```python
from build123d import *

# Parameters (mm, degrees)
F3_DEPTH = 50
F5_DEPTH = 10


with BuildPart() as f1:
    # F0 (on Front) → F1 (revolve)
    with BuildSketch(Plane.XZ):
        with BuildLine():
            Line((0, 30), (0, 15))
            Line((0, 15), (50, 15))
            Line((50, 15), (50, 50))
            Line((50, 50), (30, 50))
            Line((30, 50), (30, 35))
            ThreePointArc((30, 35), (28.5355339059, 31.4644660941), (25, 30))
            Line((25, 30), (0, 30))
        make_face()
    revolve(axis=Axis((18.1425, 0, 0), (1, 0, 0)))

    # F2 (on face) → F3 (cut)
    with BuildSketch(Plane(origin=(0, 0, 0), x_dir=(0, -1, 0), z_dir=(-1, 0, 0))):
        with BuildLine():
            ThreePointArc((15, 0), (14.9240422951, -1.5076344301), (14.6969384567, -3))
            Line((14.6969384567, -3), (18, -3))
            Line((18, -3), (18, 3))
            Line((18, 3), (14.6969384567, 3))
            ThreePointArc((14.6969384567, 3), (14.9240422951, 1.5076344301), (15, 0))
        make_face()
    extrude(amount=-F3_DEPTH, mode=Mode.SUBTRACT)

    # F4 (on face) → F5 (cut)
    with BuildSketch(Plane.YZ.offset(50)):
        with BuildLine():
            Line((-13.7477270849, 6), (-49.638694584, 6))
            ThreePointArc((-49.638694584, 6), (-50, 0), (-49.638694584, -6))
            Line((-49.638694584, -6), (-13.7477270849, -6))
            ThreePointArc((-13.7477270849, -6), (-14.3012149639, -4.5249586249), (-14.6969384567, -3))
            Line((-14.6969384567, -3), (-18, -3))
            Line((-18, -3), (-18, 3))
            Line((-18, 3), (-14.6969384567, 3))
            ThreePointArc((-14.6969384567, 3), (-14.3012149639, 4.5249586249), (-13.7477270849, 6))
        make_face()
        with BuildLine():
            ThreePointArc((50, 0), (49.9095919098, 3.0054343115), (49.638694584, 6))
            Line((49.638694584, 6), (13.7477270849, 6))
            ThreePointArc((13.7477270849, 6), (15, 0), (13.7477270849, -6))
            Line((13.7477270849, -6), (49.638694584, -6))
            ThreePointArc((49.638694584, -6), (49.9095919098, -3.0054343115), (50, 0))
        make_face()
    extrude(amount=-F5_DEPTH, mode=Mode.SUBTRACT)


solid = f1.part
```
Part model, mm, in its own coordinate system. A direction names the side the tool comes from. Coordinates: 2 decimals unless noted, no trailing zeros. Order: outer loops, then holes, each group sorted by start corner. A loop starts at its lowest first (then second) coordinate and runs counter-clockwise, first axis right, second up. Notation, with made-up numbers: (-1.5, 17.25) - (44.5, 17.25) arc R22 cw to (44.5, 45.25) - close; hole circle Ø10 at (64.25, 34.25). An arc over 180 degrees is marked (long way). Return JSON: item names as keys, results as strings. Group by question number.
Item 1: Cut at A-A (z = 0). List the corners of the cut face in (x, y).
Item 2: Drill centre lines: probe 1 along Z at (x, y) = (39, 0); probe 2 along Z at (x, y) = (13, 0); probe 3 along X at (y, z) = (-23, -34.5). Where is each one in solid material? Low to high. Write a range as from..to.
Item 3: Cut at B-B (y = 0). List the corners of the cut face in (x, z).
Item 4: Which spindle directions (+Z, -Z, +X, -X, +Y, -Y) get a long thin tool onto all of the face, cutting with end or side? Do faces 1 (the face through (0, -14, 6)), 2 (the face through (20, -16, -3)), 3 (the face through (50, -1, -28)), 4 (the face through (30, 10, -34)), 5 (the face through (45, -31, 6)). Say none if no direction does.
Item 5: Pin check, flat tips, straight feed: pin 1 (5 mm diameter, centred on x = 15, y = -10, fed in from +Z); pin 2 (6 mm diameter, centred on y = 18, z = -37, fed in from -X); pin 3 (11 mm diameter, centred on x = 44.5, y = 36, fed in from +Z); pin 4 (10 mm diameter, centred on y = 4.5, z = -33, fed in from -X). Stop position of each tip, or through.
Item 6: Cut at D-D (x = 22). List the corners of the cut face in (y, z).
Item 7: Cut at C-C (x = 45). List the corners of the cut face in (y, z).
Item 8: Pull direction Y, two halves, no side cores. Call faces 6 (the face through (39.86, -15.02, 47.69)), 7 (the face through (45, 31, -6)), 8 (the face through (25.35, 14.987, -0.617)): pulls with the +Y half, pulls with the -Y half, needs draft (parallel to the pull), parting line crosses it, or undercut.
Check values:
{
 "1": {"outline": "(0, -30) - (25, -30) arc R5 cw to (30, -35) - (30, -50) - (40, -50) - (40, -18) - (0, -18) - close; (0, 15) - (40, 15) - (40, 50) - (30, 50) - (30, 35) arc R5 cw to (25, 30) - (0, 30) - close"},
 "2": {"probe 1": "z = -50..-15, 15..50", "probe 2": "z = -30..-15, 15..30", "probe 3": "x = 30..50"},
 "3": {"outline": "(0, -30) - (25, -30) arc R5 cw to (30, -35) - (30, -50) - (50, -50) - (50, -15) - (0, -15) - close; (0, 15) - (50, 15) - (50, 50) - (30, 50) - (30, 35) arc R5 cw to (25, 30) - (0, 30) - close"},
 "4": {"face 1": "+Z, -Z, -X, +Y, -Y", "face 2": "+X, -X", "face 3": "+Z, -Z, +X, +Y, -Y", "face 4": "-X", "face 5": "+X, +Y, -Y"},
 "5": {"pin 1": "stops at z = 29.05", "pin 2": "stops at x = 30", "pin 3": "stops at z = 39.62", "pin 4": "stops at x = 0"},
 "6": {"outline": "circle Ø60 at (0, 0); hole (-18, -3) - (-14.7, -3) arc R15 ccw (long way) to (-14.7, 3) - (-18, 3) - close"},
 "7": {"outline": "(-49.64, -6) arc R50 ccw to (49.64, -6) - (13.75, -6) arc R15 cw to (-13.75, -6) - close; (-49.64, 6) - (-13.75, 6) arc R15 cw to (13.75, 6) - (49.64, 6) arc R50 ccw to start"},
 "8": {"face 6": "parting line crosses it", "face 7": "needs draft", "face 8": "undercut"}
}
